```python
from build123d import *

# Parameters (mm, degrees)
SKETCH6_W           = 1.524
SKETCH6_H           = 5.1562
CIRPATTERN1_COUNT   = 12
SKETCH7_R           = 13.81125
SKETCH7_R_2         = 6.82625
BOSS_EXTRUDE1_DEPTH = 9.525


with BuildPart() as part:
    # Sketch1 → Revolve1 (revolve)
    with BuildSketch(Plane(origin=(0, 0, 0), x_dir=(0, 0, -1), z_dir=(1, 0, 0)), mode=Mode.PRIVATE) as revolve1_sk:
        with BuildLine():
            Line((4.28625, 14.2875), (-4.28625, 14.2875))
            Line((-4.28625, 14.2875), (-4.7625, 13.81125))
            Line((-4.7625, 13.81125), (-4.7625, 10.7188))
            Line((-4.7625, 10.7188), (-2.347405, 10.7188))
            ThreePointArc((-2.347405, 10.7188), (0, 12.7), (2.347405, 10.7188))
            Line((2.347405, 10.7188), (4.7625, 10.7188))
            Line((4.7625, 10.7188), (4.7625, 13.81125))
            Line((4.7625, 13.81125), (4.28625, 14.2875))
        make_face()
    revolve(revolve1_sk.sketch.rotate(Axis((0, 0, 4.7625), (0, 0, -1)), 90), axis=Axis((0, 0, 4.7625), (0, 0, -1)))

    # Sketch6 → Revolve6 (revolve)
    with BuildSketch(Plane(origin=(0, 0, 0), x_dir=(0, 0, -1), z_dir=(1, 0, 0)), mode=Mode.PRIVATE) as revolve6_sk:
        with Locations((4.0005, 13.2969)):
            Rectangle(SKETCH6_W, SKETCH6_H)
    revolve(revolve6_sk.sketch.rotate(Axis((0, 0, -4.7625), (0, 0, 1)), 270), axis=Axis((0, 0, -4.7625), (0, 0, 1)))



with BuildPart() as body_2:
    # Sketch3 → Revolve3 (revolve)
    with BuildSketch(Plane(origin=(0, 0, 0), x_dir=(0, 0, -1), z_dir=(1, 0, 0)), mode=Mode.PRIVATE) as revolve3_sk:
        with BuildLine():
            Line((-4.7625, 6.82625), (-4.7625, 8.26135))
            Line((-4.7625, 8.26135), (-4.28625, 8.7376))
            Line((-4.28625, 8.7376), (-1.780538, 8.7376))
            ThreePointArc((-1.780538, 8.7376), (0, 7.9375), (1.780538, 8.7376))
            Line((1.780538, 8.7376), (5.88645, 8.7376))
            Line((5.88645, 8.7376), (6.3627, 8.26135))
            Line((6.3627, 8.26135), (6.3627, 6.82625))
            Line((6.3627, 6.82625), (5.88645, 6.35))
            Line((5.88645, 6.35), (-4.28625, 6.35))
            Line((-4.28625, 6.35), (-4.7625, 6.82625))
        make_face()
    revolve(revolve3_sk.sketch.rotate(Axis((0, 0, 4.7625), (0, 0, -1)), 90), axis=Axis((0, 0, 4.7625), (0, 0, -1)))


with BuildPart() as body_3:
    # Sketch4 → Revolve4 (revolve)
    with BuildSketch(Plane(origin=(0, 0, 0), x_dir=(0, 0, -1), z_dir=(1, 0, 0))):
        with BuildLine():
            Line((-2.38125, 10.31875), (2.38125, 10.31875))
            ThreePointArc((2.38125, 10.31875), (0, 12.7), (-2.38125, 10.31875))
        make_face()
    revolve(axis=Axis((0, 10.31875, 2.38125), (0, 0, -1)))


with BuildPart() as cirpattern1_1:
    # CirPattern1: pattern copy
    add(body_3.part.rotate(Axis((0, 0, 0), (0, 0, 1)), 1 * 360 / CIRPATTERN1_COUNT))


with BuildPart() as cirpattern1_2:
    # CirPattern1: pattern copy
    add(body_3.part.rotate(Axis((0, 0, 0), (0, 0, 1)), 2 * 360 / CIRPATTERN1_COUNT))


with BuildPart() as cirpattern1_3:
    # CirPattern1: pattern copy
    add(body_3.part.rotate(Axis((0, 0, 0), (0, 0, 1)), 3 * 360 / CIRPATTERN1_COUNT))


with BuildPart() as cirpattern1_4:
    # CirPattern1: pattern copy
    add(body_3.part.rotate(Axis((0, 0, 0), (0, 0, 1)), 4 * 360 / CIRPATTERN1_COUNT))


with BuildPart() as cirpattern1_5:
    # CirPattern1: pattern copy
    add(body_3.part.rotate(Axis((0, 0, 0), (0, 0, 1)), 5 * 360 / CIRPATTERN1_COUNT))


with BuildPart() as cirpattern1_6:
    # CirPattern1: pattern copy
    add(body_3.part.rotate(Axis((0, 0, 0), (0, 0, 1)), 6 * 360 / CIRPATTERN1_COUNT))


with BuildPart() as cirpattern1_7:
    # CirPattern1: pattern copy
    add(body_3.part.rotate(Axis((0, 0, 0), (0, 0, 1)), 7 * 360 / CIRPATTERN1_COUNT))


with BuildPart() as cirpattern1_8:
    # CirPattern1: pattern copy
    add(body_3.part.rotate(Axis((0, 0, 0), (0, 0, 1)), 8 * 360 / CIRPATTERN1_COUNT))


with BuildPart() as cirpattern1_9:
    # CirPattern1: pattern copy
    add(body_3.part.rotate(Axis((0, 0, 0), (0, 0, 1)), 9 * 360 / CIRPATTERN1_COUNT))


with BuildPart() as cirpattern1_10:
    # CirPattern1: pattern copy
    add(body_3.part.rotate(Axis((0, 0, 0), (0, 0, 1)), 10 * 360 / CIRPATTERN1_COUNT))


with BuildPart() as cirpattern1_11:
    # CirPattern1: pattern copy
    add(body_3.part.rotate(Axis((0, 0, 0), (0, 0, 1)), 11 * 360 / CIRPATTERN1_COUNT))


with BuildPart() as part_1:
    add(part.part)

    add(body_2.part)  # Boss-Extrude1 merges body 2

    add(body_3.part)  # Boss-Extrude1 merges body 3

    add(cirpattern1_1.part)  # Boss-Extrude1 merges CirPattern1_1

    add(cirpattern1_2.part)  # Boss-Extrude1 merges CirPattern1_2

    add(cirpattern1_3.part)  # Boss-Extrude1 merges CirPattern1_3

    add(cirpattern1_4.part)  # Boss-Extrude1 merges CirPattern1_4

    add(cirpattern1_5.part)  # Boss-Extrude1 merges CirPattern1_5

    add(cirpattern1_6.part)  # Boss-Extrude1 merges CirPattern1_6

    add(cirpattern1_7.part)  # Boss-Extrude1 merges CirPattern1_7

    add(cirpattern1_8.part)  # Boss-Extrude1 merges CirPattern1_8

    add(cirpattern1_9.part)  # Boss-Extrude1 merges CirPattern1_9

    add(cirpattern1_10.part)  # Boss-Extrude1 merges CirPattern1_10

    add(cirpattern1_11.part)  # Boss-Extrude1 merges CirPattern1_11
    # Sketch7 → Boss-Extrude1 (add)
    with BuildSketch(Plane.XY.offset(4.7625)):
        Circle(SKETCH7_R)
        Circle(SKETCH7_R_2, mode=Mode.SUBTRACT)
    extrude(amount=-BOSS_EXTRUDE1_DEPTH)


solid = part_1.part
```
Can you work these out from the model? Positions are in its coordinate system, mm. A direction names the side the tool comes from. Coordinates: 2 decimals unless noted, no trailing zeros. Use a Markdown table: item, result.
Item 1: We'd pull the mould along Y, two halves only. Please class faces 4 (the face through (-14.274, -0.628, 0.577)), 5 (the face through (-3.3, -6.3, 4.762)), 6 (the face through (-5.04, 3.86, -0.73)): released by +Y, released by -Y, zero draft, split by the parting line, or undercut.
Numbers:
| item | result |
|---|---|
| face 4 | split by the parting line |
| face 5 | zero draft |
| face 6 | undercut |
Item 2: If I drill on probe 1 along Y at (x, z) = (0, -2.5); probe 2 along Z at (x, y) = (-5, 8.5); probe 3 along Y at (x, z) = (0, -4) (3 decimals), over which ranges is the centre line in solid material (lowest first)? Write a range as from..to.
Numbers:
| item | result |
|---|---|
| probe 1 | y = -14.29..-6.35, 6.35..14.29 |
| probe 2 | z = -4.76..4.76 |
| probe 3 | y = -15.875..-6.35, 6.35..15.875 |
Item 3: Will these pins go through, and if not, where does the flat tip stop? pin 1 (1.5 mm diameter, centred on x = 8, y = 6.5, fed in from -Z); pin 2 (1.5 mm diameter, centred on x = 4.5, z = -4.5, fed in from -Y); pin 3 (1.5 mm diameter, centred on x = -5, z = -2, fed in from -Y).
Numbers:
| item | result |
|---|---|
| pin 1 | stops at z = -4.76 |
| pin 2 | stops at y = -15.43 |
| pin 3 | stops at y = -13.64 |
Item 4: For faces 1 (the face through (11.83, 8.31, -3.238)), 2 (the face through (-3.441, -15.497, -4.011)), 3 (the face through (-7, -7, -4.762)), which set-ups out of +Z, -Z, +X, -X, +Y, -Y let a thin tool reach every point of the face, with its end or its side?
Numbers:
| item | result |
|---|---|
| face 1 | +Z |
| face 2 | +Z, -Z |
| face 3 | -Z |
